Can you work these out from the model? Positions are in its coordinate system, mm. A direction names the side the tool comes from. Give positions to 0.01 mm unless a question says otherwise; leave off trailing zeros. Loops run counter-clockwise (first coordinate to the right, second up) from the corner with the lowest first, then second, coordinate; pieces in that order, holes last. Notation, with made-up numbers: (-22.75, 78) -> (9.25, 78) arc R28 ccw to (9.25, 104) -> close; hole circle Ø2 at (-15.5, 35.5). An arc over 180 degrees is marked (long way). Return JSON: item names as keys, results as strings. Group by question number.
Q1. I need wall thicknesses on line 1 along X through (y, z) = (1.4, -12); line 2 along Y through (x, z) = (4, 2.2); line 3 along Z through (x, y) = (5, 5). Which ranges of each line are inside material? Lowest first, please. Write a range as [from, to].
Q2. Suppose I cut it at C-C, the plane z = -12. Please give me the cut outline in (x, y).
Q3. Thinking about a two-plate mould opening in Z: for faces 4 (the flat face through (15, 3, -14)), 5 (the flat face through (15, 20, 3)), 6 (the cylindrical face through (3.65, 5.44, 1.52)), which applies, pulls with the +Z half, pulls with the -Z half, needs draft (parallel to the pull), parting line crosses it, or undercut?
Q4. Suppose I cut it at A-A, the plane x = 4. Please give me the cut outline in (y, z).
Q5. Which directions (+Z, -Z, +X, -X, +Y, -Y) give clear straight access to the entire face, cutting with the end or side of a thin tool? Please do faces 1 (the flat face through (15, 18, 0)), 2 (the cylindrical face through (25.792, 30.586, 1.521)), 3 (the flat face through (0, 2, -16)).
Q6. Will these pins go through, and if not, where does the flat tip stop? pin 1 (8 mm diameter, centred on x = 11.5, z = -12.5, fed in from +Y); pin 2 (2.5 mm diameter, centred on x = 26, y = 29, fed in from +Z).
Q7. Suppose I cut it at D-D, the plane z = 1.5. Please give me the cut outline in (x, y).
Q8. Suppose I cut it at B-B, the plane y = 29. Please give me the cut outline in (x, z), and give its area (3 significant figures).
```python
from build123d import *

# Parameters (mm, degrees)
SKETCH1_W           = 30
SKETCH1_H           = 30
SKETCH1_R           = 1.15
BOSS_EXTRUDE1_DEPTH = 3
SKETCH2_W           = 30
SKETCH2_H           = 3
BOSS_EXTRUDE2_DEPTH = 30
CUT_EXTRUDE1_REACH  = 55.749
SKETCH3_R           = 6
SKETCH4_W           = 30
SKETCH4_H           = 33
SKETCH4_R           = 6
BOSS_EXTRUDE3_DEPTH = 3
CUT_EXTRUDE3_REACH  = 57.48
SKETCH5_R           = 1.6


with BuildPart() as part:
    # Sketch1 → Boss-Extrude1 (new body)
    with BuildSketch(Plane(origin=(0, 0, 0), x_dir=(1, 0, 0), z_dir=(0, 1, 0))):
        with Locations((15, 15)):
            Rectangle(SKETCH1_W, SKETCH1_H)
        with Locations(Location((5.999988, 12, 0), (0, 0, 270))):
            Circle(SKETCH1_R, mode=Mode.SUBTRACT)
        with Locations(Location((23.999988, 12, 0), (0, 0, 270))):
            Circle(SKETCH1_R, mode=Mode.SUBTRACT)
    extrude(amount=BOSS_EXTRUDE1_DEPTH)

    # Sketch2 → Boss-Extrude2 (add)
    with BuildSketch(Plane(origin=(0, 3, 0), x_dir=(1, 0, 0), z_dir=(0, 1, 0))):
        with Locations((15, 28.5)):
            Rectangle(SKETCH2_W, SKETCH2_H)
    extrude(amount=BOSS_EXTRUDE2_DEPTH)

    # Sketch3 → Cut-Extrude1 (cut, up to next)
    with BuildSketch(Plane(origin=(0, 0, -30), x_dir=(-1, 0, 0), z_dir=(0, 0, -1)), mode=Mode.PRIVATE) as cut_extrude1_sk1:
        with Locations((-15, 11)):
            Circle(SKETCH3_R)
    cut_extrude1_tool1 = extrude(cut_extrude1_sk1.sketch, amount=-CUT_EXTRUDE1_REACH, mode=Mode.PRIVATE) & part.part
    add(cut_extrude1_tool1.solids().sort_by_distance((15, 11, -30))[0], mode=Mode.SUBTRACT)

    # Sketch4 → Boss-Extrude3 (add)
    with BuildSketch(Plane.XY):
        with Locations((15, 16.5)):
            Rectangle(SKETCH4_W, SKETCH4_H)
        with Locations(Location((15, 11, 0), (0, 0, 180))):
            Circle(SKETCH4_R, mode=Mode.SUBTRACT)
    extrude(amount=BOSS_EXTRUDE3_DEPTH)

    # Sketch5 → Cut-Extrude3 (cut, up to next)
    with BuildSketch(Plane.XY.offset(3), mode=Mode.PRIVATE) as cut_extrude3_sk1:
        with Locations((26, 7)):
            Circle(SKETCH5_R)
    cut_extrude3_tool1 = extrude(cut_extrude3_sk1.sketch, amount=-CUT_EXTRUDE3_REACH, mode=Mode.PRIVATE) & part.part
    # Sketch5 → Cut-Extrude3 (cut, up to next)
    with BuildSketch(Plane.XY.offset(3), mode=Mode.PRIVATE) as cut_extrude3_sk2:
        with Locations((4, 7)):
            Circle(SKETCH5_R)
    cut_extrude3_tool2 = extrude(cut_extrude3_sk2.sketch, amount=-CUT_EXTRUDE3_REACH, mode=Mode.PRIVATE) & part.part
    # Sketch5 → Cut-Extrude3 (cut, up to next)
    with BuildSketch(Plane.XY.offset(3), mode=Mode.PRIVATE) as cut_extrude3_sk3:
        with Locations((4, 29)):
            Circle(SKETCH5_R)
    cut_extrude3_tool3 = extrude(cut_extrude3_sk3.sketch, amount=-CUT_EXTRUDE3_REACH, mode=Mode.PRIVATE) & part.part
    # Sketch5 → Cut-Extrude3 (cut, up to next)
    with BuildSketch(Plane.XY.offset(3), mode=Mode.PRIVATE) as cut_extrude3_sk4:
        with Locations((26, 29)):
            Circle(SKETCH5_R)
    cut_extrude3_tool4 = extrude(cut_extrude3_sk4.sketch, amount=-CUT_EXTRUDE3_REACH, mode=Mode.PRIVATE) & part.part
    add(cut_extrude3_tool1.solids().sort_by_distance((26, 7, 3))[0], mode=Mode.SUBTRACT)
    add(cut_extrude3_tool2.solids().sort_by_distance((4, 7, 3))[0], mode=Mode.SUBTRACT)
    add(cut_extrude3_tool3.solids().sort_by_distance((4, 29, 3))[0], mode=Mode.SUBTRACT)
    add(cut_extrude3_tool4.solids().sort_by_distance((26, 29, 3))[0], mode=Mode.SUBTRACT)


solid = part.part
```
Ans:
{
 "1": {"line 1": "x = [0, 4.85], [7.15, 22.85], [25.15, 30]", "line 2": "y = [0, 5.4], [8.6, 27.4], [30.6, 33]", "line 3": "z = [-30, -27], [0, 3]"},
 "2": {"outline": "(0, 0) -> (4.85, 0) -> (4.85, 3) -> (0, 3) -> close; (7.15, 0) -> (22.85, 0) -> (22.85, 3) -> (7.15, 3) -> close; (25.15, 0) -> (30, 0) -> (30, 3) -> (25.15, 3) -> close"},
 "3": {"face 4": "undercut", "face 5": "pulls with the +Z half", "face 6": "needs draft"},
 "4": {"outline": "(0, -30) -> (33, -30) -> (33, -27) -> (3, -27) -> (3, 0) -> (5.4, 0) -> (5.4, 3) -> (0, 3) -> close; (8.6, 0) -> (27.4, 0) -> (27.4, 3) -> (8.6, 3) -> close; (30.6, 0) -> (33, 0) -> (33, 3) -> (30.6, 3) -> close"},
 "5": {"face 1": "+X, -X, +Y", "face 2": "+Z", "face 3": "+Z, -Z, -X, +Y, -Y"},
 "6": {"pin 1": "stops at y = 3", "pin 2": "stops at z = -27"},
 "7": {"outline": "(0, 0) -> (30, 0) -> (30, 33) -> (0, 33) -> close; hole circle Ø3.2 at (4, 7); hole circle Ø3.2 at (4, 29); hole circle Ø12 at (15, 11); hole circle Ø3.2 at (26, 7); hole circle Ø3.2 at (26, 29)"},
 "8": {"outline": "(0, -30) -> (30, -30) -> (30, -27) -> (0, -27) -> close; (0, 0) -> (2.4, 0) -> (2.4, 3) -> (0, 3) -> close; (5.6, 0) -> (24.4, 0) -> (24.4, 3) -> (5.6, 3) -> close; (27.6, 0) -> (30, 0) -> (30, 3) -> (27.6, 3) -> close", "area": "161 mm^2"}
}
